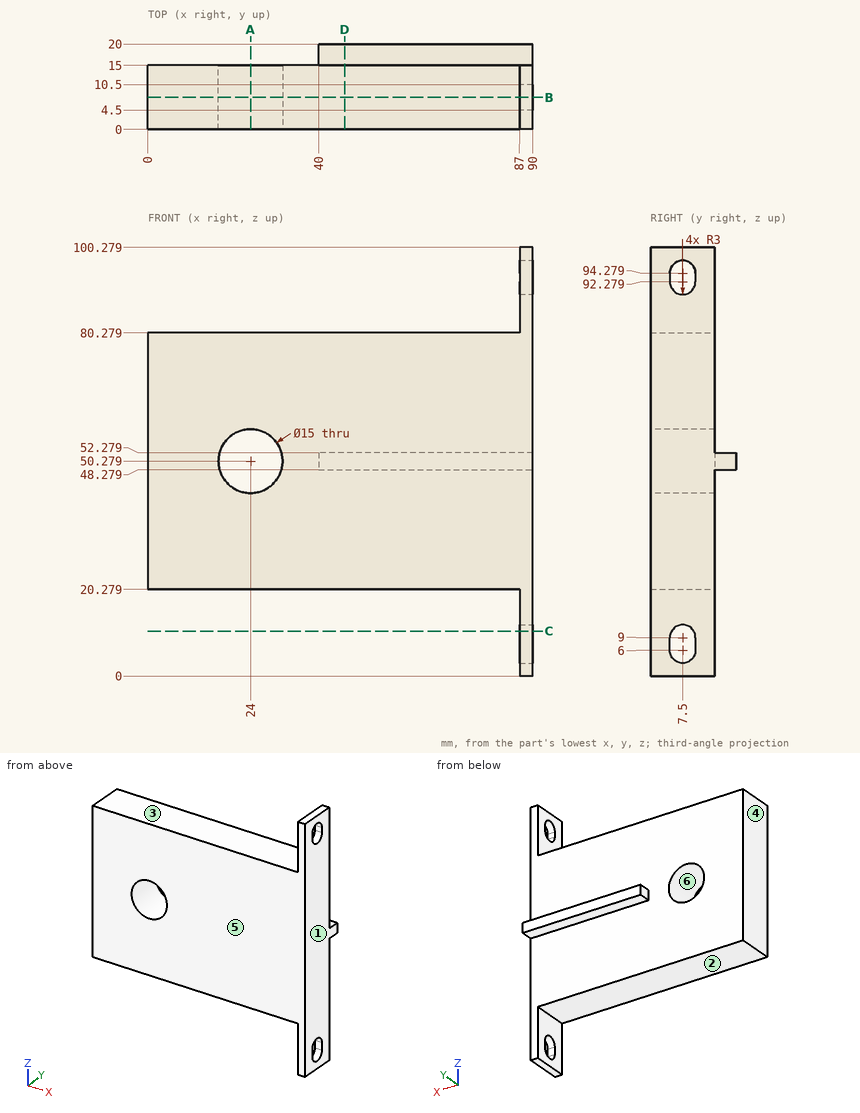
Geometry check sheet. Reference: drawing and pictorial views, mm from the part's lowest x, y, z. A direction names the side the tool comes from. Round coordinates to 2 decimals unless told otherwise and drop trailing zeros. Loops run counter-clockwise (first coordinate to the right, second up) from the corner with the lowest first, then second, coordinate; pieces in that order, holes last.
1. Sectioned sample at D-D on x = 46. Record the boundary of the cut face in (y, z).
2. Sectioned sample at C-C on z = 10.5. Record the boundary of the cut face in (x, y), and give its area (3 significant figures).
3. Scan lines: probe 1 along Z at (x, y) = (24, 10.5); probe 2 along Y at (x, z) = (71, 21.5); probe 3 along Z at (x, y) = (36.5, 3.25). Record each from-to range of solid material in increasing order.
4. Gauge pin test, flat ends, axial feed: pin 1 Ø12 at (y, z) = (7.5, 11.5) entering from -X; pin 2 Ø4 at (x, z) = (72.5, 26.5) entering from -Y; pin 3 Ø4.5 at (x, y) = (39, 6.5) entering from -Z; pin 4 Ø1 at (x, z) = (88, 93.5) entering from +Y. Record the tip position at first contact, or that the pin passes through.
5. Sectioned sample at B-B on y = 7.5. Record the boundary of the cut face in (x, z).
6. Sectioned sample at A-A on x = 24. Record the boundary of the cut face in (y, z), and give its area (3 significant figures).
7. Set-up check for the marked faces 1, 2 and 3: record each of +Z, -Z, +X, -X, +Y, -Y from which the full face is reachable in a straight line by a thin tool's end or side.
8. Mould release check, pull along X, two halves, no side actions. Record for the marked faces 4, 5 and 6: released by +X, released by -X, zero draft, split by the parting line, or undercut.
Recorded:
1. outline: (0, 20.28) - (15, 20.28) - (15, 48.28) - (20, 48.28) - (20, 52.28) - (15, 52.28) - (15, 80.28) - (0, 80.28) - close
2. outline: (87, 0) - (90, 0) - (90, 4.9) - (87, 4.9) - close; (87, 10.1) - (90, 10.1) - (90, 15) - (87, 15) - close
2. area: 29.4 mm2
3. probe 1: z = 20.28 to 42.78, 57.78 to 80.28
3. probe 2: y = 0 to 15
3. probe 3: z = 20.28 to 80.28
4. pin 1: stops at x = 87
4. pin 2: stops at y = 0
4. pin 3: stops at z = 20.28
4. pin 4: stops at y = 15
5. outline: (0, 20.28) - (87, 20.28) - (87, 12) - (90, 12) - (90, 89.28) - (87, 89.28) - (87, 80.28) - (0, 80.28) - close; (87, 0) - (90, 0) - (90, 3) - (87, 3) - close; (87, 97.28) - (90, 97.28) - (90, 100.28) - (87, 100.28) - close; hole circle Ø15 at (24, 50.28)
6. outline: (0, 20.28) - (15, 20.28) - (15, 42.78) - (0, 42.78) - close; (0, 57.78) - (15, 57.78) - (15, 80.28) - (0, 80.28) - close
6. area: 675 mm2
7. face 1: +Z, -Z, +X, +Y, -Y
7. face 2: -Z, -X, +Y, -Y
7. face 3: +Z, -X, +Y, -Y
8. face 4: released by -X
8. face 5: zero draft
8. face 6: undercut
